from build123d import *

# Parameters (mm, degrees)
SKETCH1_R      = 3.25
SKETCH1_R_2    = 1.65
MAIN_ARM_DEPTH = 10


with BuildPart() as part:
    # Sketch1 → Main Arm (new body)
    with BuildSketch(Plane.XY):
        with BuildLine():
            Line((280, 13.25), (0, 13.25))
            ThreePointArc((0, 13.25), (-13.25, 0), (0, -13.25))
            Line((0, -13.25), (280, -13.25))
            Line((280, -13.25), (280, -15))
            Line((280, -15), (320, -15))
            Line((320, -15), (320, 15))
            Line((320, 15), (280, 15))
            Line((280, 15), (280, 13.25))
        make_face()
        Circle(SKETCH1_R, mode=Mode.SUBTRACT)
        with Locations((285, 10)):
            Circle(SKETCH1_R_2, mode=Mode.SUBTRACT)
        with Locations((285, -10)):
            Circle(SKETCH1_R_2, mode=Mode.SUBTRACT)
        with BuildLine():
            Line((308, -6), (292, -6))
            ThreePointArc((292, -6), (289.878679656, -5.121320344), (289, -3))
            Line((289, -3), (289, 3))
            ThreePointArc((289, 3), (289.878679656, 5.121320344), (292, 6))
            Line((292, 6), (308, 6))
            ThreePointArc((308, 6), (310.121320344, 5.121320344), (311, 3))
            Line((311, 3), (311, -3))
            ThreePointArc((311, -3), (310.121320344, -5.121320344), (308, -6))
        make_face(mode=Mode.SUBTRACT)
        with Locations((315, 10)):
            Circle(SKETCH1_R_2, mode=Mode.SUBTRACT)
        with Locations((315, -10)):
            Circle(SKETCH1_R_2, mode=Mode.SUBTRACT)
    extrude(amount=MAIN_ARM_DEPTH)


solid = part.part
Source: CAD feature listing. Evaluate the final solid. Frame: model axes, mm. A direction names the side the tool comes from. Coordinates: 2 decimals unless noted, no trailing zeros. Order: outer loops, then holes, each group sorted by start corner. A loop starts at its lowest first (then second) coordinate and runs counter-clockwise, first axis right, second up. Notation, with made-up numbers: M 41,14.5 L 49,14.5 A25 ccw 49,52.5 Z; hole C 24.5,77.25 d6. An arc over 180 degrees is marked long. Write each question's results on one line, items separated by ' | '. Start each with the question number.
1. Section A-A, the plane z = 7.75. Return the cut outline in (x, y).
2. Section C-C, the plane x = 144. Return the cut outline in (y, z).
3. Section B-B, the plane y = 0. Return the cut outline in (x, z).
4. Draft query along X for faces 5 (the face through (320, 0, 5)), 6 (the face through (289, 0, 5)), 7 (the face through (-13.247, 0.291, 4.93)). Return one class per face: +X half, -X half, draft (parallel to the pull), parting line (faces both ways), or undercut.
5. Material intervals for L1, parallel to Y at x = 315, z = 6.5; L2, parallel to X at y = 0.5, z = 3.5; L3, parallel to X at y = -1.25, z = 7.25, sorted ascending.
6. Reachability of faces 1 (the face through (138, -13.25, 5)), 2 (the face through (300, -6, 5)), 3 (the face through (142, 13.25, 5)), 4 (the face through (151, 0, 0)) from +Z, -Z, +X, -X, +Y, -Y: full face, straight path, thin tool, end or side. Return the list, or none.
7. Pin query (flat end, axial travel): pin 1 (1.5 mm diameter, centred on x = 108, z = 4, fed in from +Y); pin 2 (3 mm diameter, centred on y = -2, z = 3.5, fed in from -X); pin 3 (6 mm diameter, centred on y = 6, z = 3.5, fed in from -X). Return the tip coordinate at first contact, or that it passes through.
Solution:
1) outline: M 0,-13.25 L 280,-13.25 L 280,-15 L 320,-15 L 320,15 L 280,15 L 280,13.25 L 0,13.25 A13.25 ccw Z; hole C 0,0 d6.5; hole C 285,-10 d3.3; hole C 285,10 d3.3; hole M 289,-3 A3 ccw 292,-6 L 308,-6 A3 ccw 311,-3 L 311,3 A3 ccw 308,6 L 292,6 A3 ccw 289,3 Z; hole C 315,-10 d3.3; hole C 315,10 d3.3
2) outline: M -13.25,0 L 13.25,0 L 13.25,10 L -13.25,10 Z
3) outline: M -13.25,0 L -3.25,0 L -3.25,10 L -13.25,10 Z; M 3.25,0 L 289,0 L 289,10 L 3.25,10 Z; M 311,0 L 320,0 L 320,10 L 311,10 Z
4) face 5: +X half | face 6: undercut | face 7: -X half
5) L1: -15 to -11.65, -8.35 to 8.35, 11.65 to 15 | L2: -13.24 to -3.21, 3.21 to 289, 311 to 320 | L3: -13.19 to -3, 3 to 289, 311 to 320
6) face 1: +Z, -Z, -X, -Y | face 2: +Z, -Z | face 3: +Z, -Z, -X, +Y | face 4: -Z, +X, -X, +Y, -Y
7) pin 1: y = 13.25 | pin 2: x = -13.24 | pin 3: x = -12.91
